Geometry check sheet. Reference: the model listing, model coordinates, mm. A direction names the side the tool comes from. Give positions to 0.01 mm unless a question says otherwise; leave off trailing zeros. Write each loop counter-clockwise with the first axis right and the second up, starting at its lowest first coordinate (ties: lowest second). Pieces come first, ordered by that corner, then holes. Notation, with made-up numbers: (56, 1) -> (79, 1) arc R29 cw to (79, 32) -> close; hole circle Ø2 at (57.5, 21.25). An arc over 180 degrees is marked (long way). One line per item, written item: value.
from build123d import *

# Parameters (mm, degrees)
BOSS_EXTRUDE1_DEPTH = 4.7625
SKETCH2_W           = 25.4
SKETCH2_H           = 3.175
BOSS_EXTRUDE2_DEPTH = 4.7625


with BuildPart() as part:
    # Sketch1 → Boss-Extrude1 (new body)
    with BuildSketch(Plane(origin=(0, 0, 0), x_dir=(1, 0, 0), z_dir=(0, 1, 0))):
        Polygon((0, 0), (-215.9, 0), (-203.2, 19.05), (0, 25.4), align=None)
    extrude(amount=BOSS_EXTRUDE1_DEPTH)

    # Sketch2 → Boss-Extrude2 (add)
    with BuildSketch(Plane(origin=(0, 4.7625, 0), x_dir=(1, 0, 0), z_dir=(0, 1, 0))):
        with Locations((-190.5, -1.5875)):
            Rectangle(SKETCH2_W, SKETCH2_H)
        with Locations((-88.9, -1.5875)):
            Rectangle(SKETCH2_W, SKETCH2_H)
    extrude(amount=-BOSS_EXTRUDE2_DEPTH)


solid = part.part
1) Scan lines: probe 1 along X at (y, z) = (4.45, 0.75); probe 2 along X at (y, z) = (0.3, -19); probe 3 along Z at (x, y) = (-53, 3.3). Record each from-to range of solid material in increasing order.
Verdict:
probe 1: -203.2 to -177.8, -101.6 to -76.2
probe 2: -203.23 to 0
probe 3: -23.74 to 0
2) Tool access check on faces 1 (the flat face through (-38, 2, 0)), 2 (the flat face through (-139, 2, 0)), 3 (the flat face through (-209, 2, 0)). Record the directions out of +Z, -Z, +X, -X, +Y, -Y that give a thin tool (end or side, any length) a straight path to the whole face; none if there is none.
Verdict:
face 1: +Z, +X, +Y, -Y
face 2: +Z, +Y, -Y
face 3: +Z, -X, +Y, -Y
3) Sectioned sample at C-C on x = -53.5. Record the cut outline in (y, z).
Verdict:
outline: (0, -23.73) -> (4.76, -23.73) -> (4.76, 0) -> (0, 0) -> close
4) Depth check by flat-ended pin: pin 1 Ø1 at (y, z) = (2, 1) entering from +X; pin 2 Ø1.5 at (x, y) = (-116.5, 1.5) entering from +Z; pin 3 Ø1.6 at (y, z) = (2, 1.5) entering from -X. Enter the tip coordinate at first touch or a pass-through.
Verdict:
pin 1: x = -76.2
pin 2: z = 0
pin 3: x = -203.2
5) Sectioned sample at B-B on z = -7.5. Record the cut outline in (x, y), plus the area to 3 significant figures.
Verdict:
outline: (-210.9, 0) -> (0, 0) -> (0, 4.76) -> (-210.9, 4.76) -> close
area: 1,000 mm^2
6) Sectioned sample at A-A on y = 3.3. Record the cut outline in (x, z) (3 decimals), plus the area to 3 significant figures.
Verdict:
outline: (-215.9, 0) -> (-203.2, -19.05) -> (0, -25.4) -> (0, 0) -> (-76.2, 0) -> (-76.2, 3.175) -> (-101.6, 3.175) -> (-101.6, 0) -> (-177.8, 0) -> (-177.8, 3.175) -> (-203.2, 3.175) -> (-203.2, 0) -> close
area: 4,800 mm^2
